```python
from build123d import *

# Parameters (mm, degrees)
F1_DEPTH  = 127
F2_W      = 25.4
F2_H      = 101.6
F3_DEPTH  = 25.4
F4_W      = 50.8
F4_H      = 25.4
F5_DEPTH  = 203.2
F6_R      = 3.81
F7_DEPTH  = 50.8
F8_R      = 3.821985
F8_R_2    = 3.81
F9_DEPTH  = 50.8
F10_W     = 38.1
F10_H     = 12.7
F11_DEPTH = 101.6
F12_R     = 3.81
F13_DEPTH = 50.8


with BuildPart() as f1:
    # F0 (on Right) → F1 (new body)
    with BuildSketch(Plane.YZ):
        with BuildLine():
            Line((-50.025108, 117.912475), (-50.025108, 29.012475))
            Line((-50.025108, 29.012475), (153.174892, 29.012475))
            ThreePointArc((153.174892, 29.012475), (57.178696, 86.271171), (-50.025108, 117.912475))
        make_face()
        with BuildLine():
            Line((153.174892, 29.012475), (-50.025108, 29.012475))
            Line((-50.025108, 29.012475), (-50.025108, -34.487525))
            Line((-50.025108, -34.487525), (-151.625108, -34.487525))
            Line((-151.625108, -34.487525), (-151.625108, -47.187525))
            ThreePointArc((-151.625108, -47.187525), (6.772136, -33.076502), (153.174892, 29.012475))
        make_face()
    extrude(amount=F1_DEPTH)

    # F2 (on face) → F3 (cut)
    with BuildSketch(Plane.XY.offset(-34.487525)):
        with Locations((50.8, -100.825108)):
            Rectangle(F2_W, F2_H)
    extrude(amount=-F3_DEPTH, mode=Mode.SUBTRACT)

    # F4 (on face) → F5 (cut)
    with BuildSketch(Plane.XZ.offset(50.025108)):
        with Locations((63.5, 79.812475)):
            Rectangle(F4_W, F4_H)
        with Locations((63.5, -9.087525)):
            Rectangle(F4_W, F4_H)
    extrude(amount=-F5_DEPTH, mode=Mode.SUBTRACT)

    # F6 (on face) → F7 (join)
    with BuildSketch(Plane.XZ.offset(151.625108)):
        with Locations((71.12, -40.837525)):
            Circle(F6_R)
        with Locations((119.38, -40.837525)):
            Circle(F6_R)
    extrude(amount=F7_DEPTH)

    # F8 (on face) → F9 (join)
    with BuildSketch(Plane.XZ.offset(151.625108)):
        with Locations((7.62, -40.837525)):
            Circle(F8_R)
        with Locations((30.48, -40.837525)):
            Circle(F8_R_2)
    extrude(amount=F9_DEPTH)

    # F10 (on face) → F11 (join)
    with BuildSketch(Plane.XZ.offset(50.025108)):
        with Locations((19.05, 111.562475)):
            Rectangle(F10_W, F10_H)
    extrude(amount=F11_DEPTH)

    # F12 (on face) → F13 (join)
    with BuildSketch(Plane.XZ.offset(151.625108)):
        with Locations((30.48, 111.562475)):
            Circle(F12_R)
        with Locations((7.62, 111.562475)):
            Circle(F12_R)
    extrude(amount=F13_DEPTH)


solid = f1.part
```
Input: part model. Units: mm. Frame: model coordinates. A direction names the side the tool comes from. Coordinates: 2 decimals unless noted, no trailing zeros. Write each loop counter-clockwise with the first axis right and the second up, starting at its lowest first coordinate (ties: lowest second). Pieces come first, ordered by that corner, then holes.
1) Section C-C on x = 119.38. Output: boundary loops of the cut face in (y, z), and give its area (3 significant figures).
2) Material intervals for line 1 along Z through (x, y) = (66.5, 29); line 2 along X through (y, z) = (-13.5, -9.5); line 3 along Z through (x, y) = (47, -38), sorted ascending.
3) Mould query, pull axis X, two halves, no side actions, for faces 1 (the flat face through (19, -100, 117.912)), 2 (the flat face through (38.1, -100, 111)), 3 (the flat face through (0, 3, 34)), 4 (the flat face through (95, -151.625, -41)). Classes: pulls with the +X half, pulls with the -X half, needs draft (parallel to the pull), parting line crosses it, or undercut.
4) Pin query (flat end, axial travel): pin 1 Ø4 at (x, z) = (97.5, -42) entering from -Y; pin 2 Ø15 at (x, y) = (58, 27) entering from +Z; pin 3 Ø3 at (x, z) = (73, 9) entering from +Y. Return the tip coordinate at first contact, or that it passes through.
5) Section D-D on y = -46. Output: boundary loops of the cut face in (x, z), and give its area (3 significant figures).
6) Set-up query: faces 5 (the flat face through (88.9, 6, 80)), 6 (the flat face through (19, -100, 105.212)), 7 (the flat face through (30, -202.425, 112)), 8 (the cylindrical face through (29.654, -176.67, 107.843)). Return all of +Z, -Z, +X, -X, +Y, -Y with unobstructed straight access to the full face (end or side cutting, diameter ignored); none if empty.
7) Section B-B on z = 71. Output: boundary loops of the cut face in (x, y).
8) Section A-A on x = 71.12. Output: boundary loops of the cut face in (y, z).
Check result:
1. outline: (-202.43, -44.65) - (-151.63, -44.65) - (-151.63, -47.19) arc R511.35 ccw to (153.17, 29.01) arc R446.82 ccw to (-50.03, 117.91) - (-50.03, -34.49) - (-151.63, -34.49) - (-151.63, -37.03) - (-202.43, -37.03) - close
1. area: 21,900 mm2
2. line 1: z = -26.98 to -21.79, 3.61 to 67.11, 92.51 to 97.48
2. line 2: x = 0 to 38.1, 88.9 to 127
2. line 3: z = -42.17 to -21.79, 3.61 to 67.11, 92.51 to 115.78
3. face 1: needs draft
3. face 2: pulls with the +X half
3. face 3: pulls with the -X half
3. face 4: undercut
4. pin 1: stops at y = -151.63
4. pin 2: stops at z = 100.76
4. pin 3: stops at y = 120.91
5. outline: (0, -43.36) - (127, -43.36) - (127, 117.24) - (0, 117.24) - close; hole (38.1, -21.79) - (88.9, -21.79) - (88.9, 3.61) - (38.1, 3.61) - close; hole (38.1, 67.11) - (88.9, 67.11) - (88.9, 92.51) - (38.1, 92.51) - close
5. area: 17,800 mm2
6. face 5: +Y, -Y
6. face 6: +X, -X, -Y
6. face 7: +Z, -Z, +X, -X, -Y
6. face 8: -Y
7. outline: (0, -50.03) - (38.1, -50.03) - (38.1, 88.67) - (0, 88.67) - close; (88.9, -50.03) - (127, -50.03) - (127, 88.67) - (88.9, 88.67) - close
8. outline: (-202.43, -44.65) - (-151.63, -44.65) - (-151.63, -47.19) arc R511.35 ccw to (45.4, -21.79) - (-50.03, -21.79) - (-50.03, -34.49) - (-151.63, -34.49) - (-151.63, -37.03) - (-202.43, -37.03) - close; (-50.03, 3.61) - (107.33, 3.61) arc R511.35 ccw to (153.17, 29.01) arc R446.82 ccw to (95.78, 67.11) - (-50.03, 67.11) - close; (-50.03, 92.51) - (42.18, 92.51) arc R446.82 ccw to (-50.03, 117.91) - close
